```python
from build123d import *

# Parameters (mm, degrees)
SKETCH1_W           = 225
SKETCH1_H           = 145
SKETCH1_R           = 1.5
SKETCH1_R_2         = 2
SKETCH1_W_2         = 40
SKETCH1_H_2         = 72
BOSS_EXTRUDE1_DEPTH = 2
SKETCH3_R           = 1.5
CUT_EXTRUDE1_DEPTH  = 10
FILLET3_R           = 3
FILLET4_R           = 3
FILLET5_R           = 3.5


with BuildPart() as part:
    # Sketch1 → Boss-Extrude1 (new body)
    with BuildSketch(Plane(origin=(0, 0, 0), x_dir=(1, 0, 0), z_dir=(0, 1, 0))):
        with Locations((16.5, 0)):
            Rectangle(SKETCH1_W, SKETCH1_H)
        with Locations(Location((-85, 69, 0), (0, 0, 270))):
            Circle(SKETCH1_R, mode=Mode.SUBTRACT)
        with Locations(Location((-65, 69, 0), (0, 0, 270))):
            Circle(SKETCH1_R, mode=Mode.SUBTRACT)
        with Locations(Location((-85, -69, 0), (0, 0, 90))):
            Circle(SKETCH1_R, mode=Mode.SUBTRACT)
        with Locations(Location((-65, -69, 0), (0, 0, 90))):
            Circle(SKETCH1_R, mode=Mode.SUBTRACT)
        with Locations(Location((45, 20, 0), (0, 0, 270))):
            Circle(SKETCH1_R_2, mode=Mode.SUBTRACT)
        with Locations(Location((45, -20, 0), (0, 0, 270))):
            Circle(SKETCH1_R_2, mode=Mode.SUBTRACT)
        with Locations(Location((-80, 69, 0), (0, 0, 270))):
            Circle(SKETCH1_R, mode=Mode.SUBTRACT)
        with Locations(Location((-70, 69, 0), (0, 0, 270))):
            Circle(SKETCH1_R, mode=Mode.SUBTRACT)
        with Locations(Location((-80, -69, 0), (0, 0, 270))):
            Circle(SKETCH1_R, mode=Mode.SUBTRACT)
        with Locations(Location((-70, -69, 0), (0, 0, 270))):
            Circle(SKETCH1_R, mode=Mode.SUBTRACT)
        with Locations(Location((78.5, -40, 0), (0, 0, 270))):
            Circle(SKETCH1_R, mode=Mode.SUBTRACT)
        with Locations(Location((111.5, -40, 0), (0, 0, 270))):
            Circle(SKETCH1_R, mode=Mode.SUBTRACT)
        with Locations(Location((111.5, 40, 0), (0, 0, 270))):
            Circle(SKETCH1_R, mode=Mode.SUBTRACT)
        with Locations(Location((78.5, 40, 0), (0, 0, 270))):
            Circle(SKETCH1_R, mode=Mode.SUBTRACT)
        with Locations(Location((-92.5, -69, 0), (0, 0, 270))):
            Circle(SKETCH1_R, mode=Mode.SUBTRACT)
        with Locations(Location((-57.5, -69, 0), (0, 0, 270))):
            Circle(SKETCH1_R, mode=Mode.SUBTRACT)
        with Locations(Location((-92.5, 69, 0), (0, 0, 270))):
            Circle(SKETCH1_R, mode=Mode.SUBTRACT)
        with Locations(Location((-57.5, 69, 0), (0, 0, 270))):
            Circle(SKETCH1_R, mode=Mode.SUBTRACT)
        with Locations((91.5, 0)):
            Rectangle(SKETCH1_W_2, SKETCH1_H_2, mode=Mode.SUBTRACT)
    extrude(amount=BOSS_EXTRUDE1_DEPTH)

    # Sketch3 → Cut-Extrude1 (cut)
    with BuildSketch(Plane(origin=(0, 2, 0), x_dir=(1, 0, 0), z_dir=(0, 1, 0))):
        with BuildLine():
            Line((-54, -72.5), (35.500000021, -72.5))
            ThreePointArc((35.500000021, -72.5), (33.025126273, -71.474873741), (32, -69))
            Line((32, -69), (32, -65))
            Line((32, -65), (-54, -65))
            Line((-54, -65), (-54, -72.5))
        make_face()
        with BuildLine():
            Line((122, -69), (122, -65))
            Line((122, -65), (39, -65))
            Line((39, -65), (39, -69))
            ThreePointArc((39, -69), (37.974873741, -71.474873727), (35.500000021, -72.5))
            Line((35.500000021, -72.5), (125.499999987, -72.5))
            ThreePointArc((125.499999987, -72.5), (123.025126261, -71.47487373), (122, -69))
        make_face()
        with BuildLine():
            Line((35.5, 72.5), (-54, 72.5))
            Line((-54, 72.5), (-54, 65))
            Line((-54, 65), (32, 65))
            Line((32, 65), (32, 69))
            ThreePointArc((32, 69), (33.025126266, 71.474873734), (35.5, 72.5))
        make_face()
        with BuildLine():
            Line((125.5, 72.5), (35.5, 72.5))
            ThreePointArc((35.5, 72.5), (37.974873734, 71.474873734), (39, 69))
            Line((39, 69), (39, 65))
            Line((39, 65), (122, 65))
            Line((122, 65), (122, 69))
            ThreePointArc((122, 69), (123.025126266, 71.474873734), (125.5, 72.5))
        make_face()
        with BuildLine():
            Line((129, 72.5), (125.5, 72.5))
            ThreePointArc((125.5, 72.5), (127.974873734, 71.474873734), (129, 69))
            Line((129, 69), (129, 72.5))
        make_face()
        with Locations(Location((125.5, 69, 0), (0, 0, 270))):
            Circle(SKETCH3_R)
        with Locations(Location((35.5, 69, 0), (0, 0, 270))):
            Circle(SKETCH3_R)
        with Locations(Location((35.5, -69, 0), (0, 0, 270))):
            Circle(SKETCH3_R)
        with BuildLine():
            Line((129, -72.5), (129, -69))
            ThreePointArc((129, -69), (127.97487373, -71.474873739), (125.499999987, -72.5))
            Line((125.499999987, -72.5), (129, -72.5))
        make_face()
        with Locations(Location((125.5, -69, 0), (0, 0, 270))):
            Circle(SKETCH3_R)
    extrude(amount=-CUT_EXTRUDE1_DEPTH, mode=Mode.SUBTRACT)

    # Fillet3
    fillet3_edges = [part.edges().sort_by_distance(p)[0] for p in [
        (71.5, 1, -36),
        (71.5, 1, 36),
        (111.5, 1, 36),
        (111.5, 1, -36),
    ]]
    fillet(fillet3_edges, radius=FILLET3_R)

    # Fillet4
    fillet4_edges = [part.edges().sort_by_distance(p)[0] for p in [
        (-54, 1, 65),
        (32, 1, 65),
        (122, 1, -65),
        (39, 1, -65),
        (39, 1, 65),
        (122, 1, 65),
        (32, 1, -65),
        (-54, 1, -65),
    ]]
    fillet(fillet4_edges, radius=FILLET4_R)

    # Fillet5
    fillet5_edges = [part.edges().sort_by_distance(p)[0] for p in [
        (-54, 1, 72.5),
        (-54, 1, -72.5),
        (-96, 1, -72.5),
        (-96, 1, 72.5),
    ]]
    fillet(fillet5_edges, radius=FILLET5_R)


solid = part.part
```
For this review, take the finished solid that the model builds, in its own axes (mm). Give positions to 0.01 mm unless a question says otherwise; leave off trailing zeros. Write each loop counter-clockwise with the first axis right and the second up, starting at its lowest first coordinate (ties: lowest second). Pieces come first, ordered by that corner, then holes.
Item 1: Take a section at C-C (x = 13). Give the boundary of the cut face in (y, z), and give its area (3 significant figures).
Item 2: Take a section at A-A (x = 105.5). Give the boundary of the cut face in (y, z), and give its area (3 significant figures).
Item 3: Insertion check: P1, Ø1, axis at x = 92.5, y = 1, coming from the +Z side; P2, Ø0.6, axis at x = -18.5, y = 1.5, coming from the -Z side. Each pin has a flat end and moves straight along its axis. Give the tip position at first contact, or say it passes through.
Item 4: Wall thickness on probe 1 along Z at (x, y) = (-80, 0.5); probe 2 along X at (y, z) = (1.15, -17); probe 3 along Z at (x, y) = (105, 0.45): over which ranges is each line inside the solid? List them lowest first.
Item 5: Take a section at B-B (y = 1.35). Give the number of separate pieces and of enclosed holes in the cut face, and give its area (3 significant figures).
Established:
1. outline: (0, -65) - (2, -65) - (2, 65) - (0, 65) - close
1. area: 260 mm2
2. outline: (0, -65) - (2, -65) - (2, -36) - (0, -36) - close; (0, 36) - (2, 36) - (2, 65) - (0, 65) - close
2. area: 116 mm2
3. P1: stops at z = 65
3. P2: stops at z = -65
4. probe 1: z = -72.5 to -70.5, -67.5 to 67.5, 70.5 to 72.5
4. probe 2: x = -96 to 71.5, 111.5 to 129
4. probe 3: z = -65 to -36, 36 to 65
5. separate pieces: 1
5. enclosed holes: 23
5. area: 27,000 mm2
